from build123d import *

# Parameters (mm, degrees)
SKETCH_1_R               = 50
SKETCH_1_R_2             = 9
EXTRUDE_1_DEPTH          = 50
SKETCH_2_R               = 2.5
CUT_EXTRUDE_1_DEPTH      = 87.602540378
PATTERN_CIRCULAR_1_COUNT = 6


with BuildPart() as part:
    # Эскиз1 → Бобышка-Вытянуть1 (new body)
    with BuildSketch(Plane.XY):
        Circle(SKETCH_1_R)
        Circle(SKETCH_1_R_2, mode=Mode.SUBTRACT)
    extrude(amount=EXTRUDE_1_DEPTH)

    # Эскиз2 → Вырез-Вытянуть1 (cut, symmetric)
    with BuildSketch(Plane.XY.offset(50)):
        with Locations((23.75, 0)):
            Circle(SKETCH_2_R)
    cut_extrude_1 = extrude(amount=CUT_EXTRUDE_1_DEPTH, both=True, mode=Mode.SUBTRACT)

    # Круговой массив1: Вырез-Вытянуть1 ×6 about axis
    pattern_circular_1_axis = Axis((0, 0, 0), (0, 0, 1))
    for i in range(1, PATTERN_CIRCULAR_1_COUNT):
        add(cut_extrude_1.rotate(pattern_circular_1_axis, i * 360 / PATTERN_CIRCULAR_1_COUNT), mode=Mode.SUBTRACT)


solid = part.part
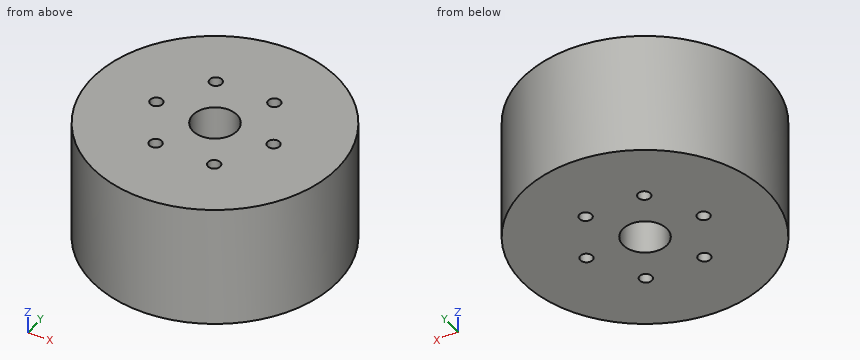
Can you work these out from the model? Positions are in its coordinate system, mm. Give positions to 0.01 mm unless a question says otherwise; leave off trailing zeros. Loops run counter-clockwise (first coordinate to the right, second up) from the corner with the lowest first, then second, coordinate; pieces in that order, holes last. Notation, with made-up numbers: (-23, 86) - (28, 86) arc R14 ccw to (28, 100) - close; hole circle Ø11 at (76.5, 80). An arc over 180 degrees is marked (long way). Return JSON: item names as keys, results as strings.
1. I want a section at A-A on y = 0. Please give me the cut outline in (x, z).
Output values:
{"outline": "(-50, 0) - (-26.25, 0) - (-26.25, 50) - (-50, 50) - close; (-21.25, 0) - (-9, 0) - (-9, 50) - (-21.25, 50) - close; (9, 0) - (21.25, 0) - (21.25, 50) - (9, 50) - close; (26.25, 0) - (50, 0) - (50, 50) - (26.25, 50) - close"}
2. If I drill on line 1 (X direction, y = 5.5, z = 25); line 2 (X direction, y = 3, z = 44.5); line 3 (X direction, y = -1, z = 15), over which ranges is the centre line in solid material (lowest first)?
Output values:
{"line 1": "x = -49.7 to -7.12, 7.12 to 49.7", "line 2": "x = -49.91 to -8.49, 8.49 to 49.91", "line 3": "x = -49.99 to -26.04, -21.46 to -8.94, 8.94 to 21.46, 26.04 to 49.99"}
3. I want a section at D-D on x = 23.75. Please give me the cut outline in (y, z).
Output values:
{"outline": "(-44, 0) - (-2.5, 0) - (-2.5, 50) - (-44, 50) - close; (2.5, 0) - (44, 0) - (44, 50) - (2.5, 50) - close"}
4. I want a section at C-C on z = 40. Please give me the cut outline in (x, y) (3 decimals).
Output values:
{"outline": "circle Ø100 at (0, 0); hole circle Ø5 at (-23.75, 0); hole circle Ø5 at (-11.875, -20.568); hole circle Ø5 at (-11.875, 20.568); hole circle Ø18 at (0, 0); hole circle Ø5 at (11.875, -20.568); hole circle Ø5 at (11.875, 20.568); hole circle Ø5 at (23.75, 0)"}
5. I'm going to push flat-ended pins straight in: pin 1 Ø1.5 at (x, z) = (-14, 27.5) entering from +Y; pin 2 Ø3 at (x, y) = (-11.88, -20.57) entering from -Z; pin 3 Ø1.5 at (x, z) = (33.5, 43.5) entering from +Y; pin 4 Ø1.5 at (x, z) = (-10, 29) entering from -Y. Where does each tip first touch, or does it pass through?
Output values:
{"pin 1": "stops at y = 48.21", "pin 2": "passes through", "pin 3": "stops at y = 37.78", "pin 4": "stops at y = -49.14"}
6. I want a section at B-B on x = 0. Please give me the cut outline in (y, z), and give its area (3 significant figures).
Output values:
{"outline": "(-50, 0) - (-9, 0) - (-9, 50) - (-50, 50) - close; (9, 0) - (50, 0) - (50, 50) - (9, 50) - close", "area": "4,100 mm²"}
